```python
from build123d import *

# Parameters (mm, degrees)
SKETCH1_R                       = 3
BOSS_EXTRUDE1_DEPTH             = 42
M4_CLEARANCE_HOLE1_D            = 4.5
TAP_DRILL_FOR_M4X0_7_TAP1_D     = 3.3
TAP_DRILL_FOR_M4X0_7_TAP1_DEPTH = 5.08
TAP_DRILL_FOR_M4X0_7_TAP1_TIP   = 0.991420021


with BuildPart() as part:
    # Sketch1 → Boss-Extrude1 (new body)
    with BuildSketch(Plane.XY):
        Polygon((-12.5, -9.5), (-9.5, -12.5), (-4, -12.5), (-4, -9.5), (5, -9.5), (5, -11), (3.55, -11), (3.55, -12.5), (9.5, -12.5), (12.5, -9.5), (12.5, 9.5), (9.5, 12.5), (3.55, 12.5), (3.55, 11), (5, 11), (5, 9.5), (-4, 9.5), (-4, 12.5), (-9.5, 12.5), (-12.5, 9.5), (-12.5, 3.55), (-11, 3.55), (-11, 5), (-9.5, 5), (-9.5, -4), (-12.5, -4), align=None)
        with Locations(Location((0, 0, 0), (0, 0, 180))):
            Circle(SKETCH1_R, mode=Mode.SUBTRACT)
    extrude(amount=BOSS_EXTRUDE1_DEPTH)

    # M4 Clearance Hole1 (through all)
    with Locations(Plane.XY.offset(42)):
        with Locations((6.560660172, 6.560660172), (-6.560660172, -6.560660172)):
            Hole(M4_CLEARANCE_HOLE1_D / 2)

    # Tap Drill for M4x0.7 Tap1
    with Locations(Plane(origin=(12.5, 0, 0), x_dir=(0, 0, -1), z_dir=(1, 0, 0))):
        with Locations((-35.5, -6), (-6.5, -6)):
            Hole(TAP_DRILL_FOR_M4X0_7_TAP1_D / 2, depth=TAP_DRILL_FOR_M4X0_7_TAP1_DEPTH)
            with Locations((0, 0, -(TAP_DRILL_FOR_M4X0_7_TAP1_DEPTH + TAP_DRILL_FOR_M4X0_7_TAP1_TIP / 2))):  # 118° drill point
                Cone(0, TAP_DRILL_FOR_M4X0_7_TAP1_D / 2, TAP_DRILL_FOR_M4X0_7_TAP1_TIP, mode=Mode.SUBTRACT)


solid = part.part
```
Verification items for the finished model (mm, model axes). A direction names the side the tool comes from. Round coordinates to 2 decimals unless told otherwise and drop trailing zeros. Loops run counter-clockwise (first coordinate to the right, second up) from the corner with the lowest first, then second, coordinate; pieces in that order, holes last. Notation, with made-up numbers: (9, 4) -> (27, 4) arc R13 cw to (27, 13) -> close; hole circle Ø9 at (54, 10.25). An arc over 180 degrees is marked (long way). Answer as a JSON object with one key per item and string values.
Q1. Go/stop test with flat-tipped pins: P1, Ø1.5, axis at x = -11, z = 15.5, coming from the +Y side; P2, Ø3.5, axis at x = 0, y = 0, coming from the +Z side; P3, Ø10, axis at x = -0.5, y = 2.5, coming from the +Z side; P4, Ø1.2, axis at y = -10.5, z = 26, coming from the -X side. Record where each tip stops, or that it passes through.
Data:
{"P1": "stops at y = 11.75", "P2": "passes through", "P3": "stops at z = 42", "P4": "stops at x = -12.1"}
Q2. Draft check along Z on faces 6 (the flat face through (3, -3, 0)), 7 (the flat face through (3, -3, 42)), 8 (the cylindrical face through (9.92, -7, 5.19)), 9 (the flat face through (12.5, 0, 21)). Enter one of: pulls with the +Z half, pulls with the -Z half, needs draft (parallel to the pull), parting line crosses it, or undercut.
Data:
{"face 6": "pulls with the -Z half", "face 7": "pulls with the +Z half", "face 8": "undercut", "face 9": "needs draft"}
Q3. Scan lines: line 1 (Z direction, x = 9.3, y = -6); line 2 (X direction, y = 4, z = 30); line 3 (Y direction, x = -6.75, z = 15.5). Record each from-to range of solid material in increasing order. Write a range as from..to.
Data:
{"line 1": "z = 0..4.85, 8.15..33.85, 37.15..42", "line 2": "x = -12.5..-11, -9.5..12.5", "line 3": "y = -12.5..-8.8, -4.32..12.5"}
Q4. Access from +Z, -Z, +X, -X, +Y, -Y to the whole of each face (thin tool, end or side, straight path). Record for faces 1 (the cylindrical face through (9.92, -5.93, 33.85)), 2 (the flat face through (3.55, -12, 21)), 3 (the flat face through (-11, -4, 21)), 4 (the flat face through (1, 9.5, 21)), 5 (the flat face through (3.55, 12, 21)).
Data:
{"face 1": "+X", "face 2": "+Z, -Z, -Y", "face 3": "+Z, -Z, -X", "face 4": "+Z, -Z", "face 5": "+Z, -Z, +Y"}
Q5. Section check C-C (z = 20). State how many separate pieces and enclosed holes the cut face has, then the cut area to 3 significant figures.
Data:
{"separate pieces": "1", "enclosed holes": "3", "area": "472 mm2"}
Q6. Section check A-A (y = 0). Record the boundary of the cut face in (x, z).
Data:
{"outline": "(-9.5, 0) -> (-3, 0) -> (-3, 42) -> (-9.5, 42) -> close; (3, 0) -> (12.5, 0) -> (12.5, 42) -> (3, 42) -> close"}
Q7. Section check B-B (x = -1.25). Record the boundary of the cut face in (y, z), then the cut area to 3 significant figures.
Data:
{"outline": "(-9.5, 0) -> (-2.73, 0) -> (-2.73, 42) -> (-9.5, 42) -> close; (2.73, 0) -> (9.5, 0) -> (9.5, 42) -> (2.73, 42) -> close", "area": "569 mm2"}
